from build123d import *

# Parameters (mm, degrees)
BOSS_EXTRUDE1_DEPTH = 12.7
SKETCH2_R           = 7.9375
CUT_EXTRUDE1_DEPTH  = 25.4
CUT_EXTRUDE2_DEPTH  = 15.24
CUT_EXTRUDE4_DEPTH  = 12.7
CUT_EXTRUDE3_DEPTH  = 12.7
FILLET4_R           = 3.81
CUT_EXTRUDE8_REACH  = 306.459
SKETCH10_R          = 3.302
CUT_EXTRUDE9_DEPTH  = 12.7
CUT_EXTRUDE10_DEPTH = 15.24
FILLET8_R           = 2.54
FILLET9_R           = 3.81
CUT_EXTRUDE11_DEPTH = 12.7
BOSS_EXTRUDE2_DEPTH = 12.7
SKETCH16_R          = 5.08
SKETCH16_R_2        = 2.54
BOSS_EXTRUDE3_DEPTH = 12.7
SKETCH17_R          = 2.54
CUT_EXTRUDE12_DEPTH = 12.7
CUT_EXTRUDE13_DEPTH = 12.7
BOSS_EXTRUDE4_DEPTH = 12.7


with BuildPart() as part:
    # Sketch1 → Boss-Extrude1 (new body)
    with BuildSketch(Plane.XY):
        with BuildLine():
            Line((22.605250022, 67.052290313), (98.805250022, 67.052290313))
            Line((98.805250022, 67.052290313), (98.805250022, 155.952290313))
            Line((98.805250022, 155.952290313), (-49.161223166, 287.699993186))
            ThreePointArc((-49.161223166, 287.699993186), (-96.236474745, 204.218681994), (-40.152034083, 126.502891159))
            Line((-40.152034083, 126.502891159), (22.605250022, 130.274128502))
            Line((22.605250022, 130.274128502), (22.605250022, 67.052290313))
        make_face()
    extrude(amount=BOSS_EXTRUDE1_DEPTH)

    # Sketch2 → Cut-Extrude1 (cut)
    with BuildSketch(Plane.XY.offset(12.7)):
        with Locations((-7.239749978, 209.038290313)):
            Circle(SKETCH2_R)
    extrude(amount=-CUT_EXTRUDE1_DEPTH, mode=Mode.SUBTRACT)

    # Sketch3 → Cut-Extrude2 (cut)
    with BuildSketch(Plane.XY.offset(12.7)):
        Polygon((41.655250022, 70.862290313), (41.655250022, 83.562290313), (60.705250022, 108.644790313), (79.755250022, 83.562290313), (79.755250022, 70.862290313), align=None)
        Polygon((26.415250022, 86.102290313), (39.115250022, 86.102290313), (57.847750022, 111.502290313), (39.115250022, 136.902290313), (26.415250022, 136.902290313), align=None)
        Polygon((94.995250022, 86.102290313), (82.295250022, 86.102290313), (63.562750022, 111.502290313), (82.295250022, 136.902290313), (94.995250022, 136.902290313), align=None)
        Polygon((41.655250022, 152.142290313), (41.655250022, 139.442290313), (60.705250022, 114.359790313), (79.755250022, 139.442290313), (79.755250022, 152.142290313), align=None)
    extrude(amount=-CUT_EXTRUDE2_DEPTH, mode=Mode.SUBTRACT)

    # Sketch5 → Cut-Extrude4 (cut)
    with BuildSketch(Plane.XY.offset(12.7)):
        with BuildLine():
            Line((-0.75941726, 237.80168728), (-42.818220106, 275.250377791))
            ThreePointArc((-42.818220106, 275.250377791), (-82.302366375, 205.259118271), (-35.720460653, 139.777057558))
            Line((-35.720460653, 139.777057558), (-14.124378137, 196.518923262))
            ThreePointArc((-14.124378137, 196.518923262), (-21.320643715, 206.617321953), (-17.910409102, 218.539326578))
            Line((-17.910409102, 218.539326578), (-0.75941726, 237.80168728))
        make_face()
        with BuildLine():
            Line((-5.26797782, 223.189077245), (3.983097906, 233.579004496))
            Line((3.983097906, 233.579004496), (15.365134305, 223.444565813))
            Line((15.365134305, 223.444565813), (6.380422315, 213.353792944))
            ThreePointArc((6.380422315, 213.353792944), (1.977645927, 219.954895508), (-5.26797782, 223.189077245))
        make_face()
        Polygon((20.700250022, 149.602290313), (-10.546123475, 195.20949671), (-35.128405597, 130.621646119), (20.700250022, 133.976525379), align=None)
    extrude(amount=-CUT_EXTRUDE4_DEPTH, mode=Mode.SUBTRACT)

    # Sketch4 → Cut-Extrude3 (cut)
    with BuildSketch(Plane.XY.offset(12.7)):
        Polygon((20.968161353, 155.952290313), (-3.903453401, 192.254898923), (20.952186028, 220.170386062), (68.306030681, 178.007049188), (68.306030681, 155.952290313), align=None)
        Polygon((91.166030681, 155.952290313), (70.846030681, 155.952290313), (70.846030681, 174.044992428), align=None)
    extrude(amount=-CUT_EXTRUDE3_DEPTH, mode=Mode.SUBTRACT)

    # Fillet4
    fillet4_edges = [part.edges().sort_by_distance(p)[0] for p in [
        (-10.546123475, 195.20949671, 6.35),
        (20.968161353, 155.952290313, 6.35),
    ]]
    fillet(fillet4_edges, radius=FILLET4_R)

    # Sketch10 → Cut-Extrude8 (cut, up to next)
    with BuildSketch(Plane.XY.offset(12.7), mode=Mode.PRIVATE) as cut_extrude8_sk1:
        with Locations((32.765250022, 77.212290313)):
            Circle(SKETCH10_R)
    cut_extrude8_tool1 = extrude(cut_extrude8_sk1.sketch, amount=-CUT_EXTRUDE8_REACH, mode=Mode.PRIVATE) & part.part
    # Sketch10 → Cut-Extrude8 (cut, up to next)
    with BuildSketch(Plane.XY.offset(12.7), mode=Mode.PRIVATE) as cut_extrude8_sk2:
        with Locations((32.765250022, 145.792290313)):
            Circle(SKETCH10_R)
    cut_extrude8_tool2 = extrude(cut_extrude8_sk2.sketch, amount=-CUT_EXTRUDE8_REACH, mode=Mode.PRIVATE) & part.part
    # Sketch10 → Cut-Extrude8 (cut, up to next)
    with BuildSketch(Plane.XY.offset(12.7), mode=Mode.PRIVATE) as cut_extrude8_sk3:
        with Locations((88.645250022, 145.792290313)):
            Circle(SKETCH10_R)
    cut_extrude8_tool3 = extrude(cut_extrude8_sk3.sketch, amount=-CUT_EXTRUDE8_REACH, mode=Mode.PRIVATE) & part.part
    # Sketch10 → Cut-Extrude8 (cut, up to next)
    with BuildSketch(Plane.XY.offset(12.7), mode=Mode.PRIVATE) as cut_extrude8_sk4:
        with Locations((88.645250022, 77.212290313)):
            Circle(SKETCH10_R)
    cut_extrude8_tool4 = extrude(cut_extrude8_sk4.sketch, amount=-CUT_EXTRUDE8_REACH, mode=Mode.PRIVATE) & part.part
    add(cut_extrude8_tool1.solids().sort_by_distance((32.76525, 77.21229, 12.7))[0], mode=Mode.SUBTRACT)
    add(cut_extrude8_tool2.solids().sort_by_distance((32.76525, 145.79229, 12.7))[0], mode=Mode.SUBTRACT)
    add(cut_extrude8_tool3.solids().sort_by_distance((88.64525, 145.79229, 12.7))[0], mode=Mode.SUBTRACT)
    add(cut_extrude8_tool4.solids().sort_by_distance((88.64525, 77.21229, 12.7))[0], mode=Mode.SUBTRACT)

    # Sketch11 → Cut-Extrude9 (cut)
    with BuildSketch(Plane.XY.offset(12.7)):
        with BuildLine():
            Line((-53.699981311, 142.099051734), (-44.964720503, 136.910524137))
            Line((-44.964720503, 136.910524137), (-50.020521881, 123.626837035))
            Line((-50.020521881, 123.626837035), (-66.867730014, 134.987909964))
            ThreePointArc((-66.867730014, 134.987909964), (-63.911601381, 136.652385518), (-60.829717039, 138.070540751))
            ThreePointArc((-60.829717039, 138.070540751), (-57.16682096, 139.911304034), (-53.699981311, 142.099051734))
        make_face()
    extrude(amount=-CUT_EXTRUDE9_DEPTH, mode=Mode.SUBTRACT)

    # Sketch13 → Cut-Extrude10 (cut)
    with BuildSketch(Plane.XY.offset(12.7)):
        with BuildLine():
            Line((-50.310364079, 281.9212995), (-42.818220106, 275.250377791))
            Line((-42.818220106, 275.250377791), (-55.824588323, 151.935966869))
            Line((-55.824588323, 151.935966869), (-61.138010202, 143.754384394))
            ThreePointArc((-61.138010202, 143.754384394), (-91.639185725, 215.652371712), (-50.310364079, 281.9212995))
        make_face()
    extrude(amount=-CUT_EXTRUDE10_DEPTH, mode=Mode.SUBTRACT)

    # Fillet8
    fillet8_edges = [part.edges().sort_by_distance(p)[0] for p in [
        (-60.829717039, 138.070540751, 6.35),
        (-61.138010202, 143.754384394, 6.35),
    ]]
    fillet(fillet8_edges, radius=FILLET8_R)

    # Fillet9
    fillet9_edges = [part.edges().sort_by_distance(p)[0] for p in [
        (-55.824588323, 151.935966869, 6.35),
    ]]
    fillet(fillet9_edges, radius=FILLET9_R)

    # Sketch14 → Cut-Extrude11 (cut)
    with BuildSketch(Plane.XY.offset(12.7)):
        Polygon((-0.75941726, 237.80168728), (-90.284904, 256.297301642), (-56.503441725, 294.237422972), (2.618728967, 241.595699413), align=None)
    extrude(amount=-CUT_EXTRUDE11_DEPTH, mode=Mode.SUBTRACT)

    # Sketch15 → Boss-Extrude2 (add)
    with BuildSketch(Plane.XY.offset(12.7)):
        Polygon((2.618728967, 241.595699413), (-83.695447283, 254.935945734), (-84.471371658, 249.915553183), (-1.404499457, 237.07719239), align=None)
    extrude(amount=-BOSS_EXTRUDE2_DEPTH)

    # Sketch16 → Boss-Extrude3 (add)
    with BuildSketch(Plane.XY.offset(12.7)):
        with Locations((-81.616731922, 249.474355701)):
            Circle(SKETCH16_R)
        with Locations((-81.616731922, 249.474355701)):
            Circle(SKETCH16_R_2, mode=Mode.SUBTRACT)
    extrude(amount=-BOSS_EXTRUDE3_DEPTH)

    # Sketch17 → Cut-Extrude12 (cut)
    with BuildSketch(Plane.XY.offset(12.7)):
        with Locations((-81.616731922, 249.474355701)):
            Circle(SKETCH17_R)
    extrude(amount=-CUT_EXTRUDE12_DEPTH, mode=Mode.SUBTRACT)

    # Sketch18 → Cut-Extrude13 (cut)
    with BuildSketch(Plane.XY.offset(12.7)):
        Polygon((-76.596339371, 248.698431326), (1.977645927, 219.954895508), (91.166030681, 155.952290313), (97.725254163, 155.952290313), (11.18255191, 258.990487802), (-76.596339371, 256.904187462), align=None)
    extrude(amount=-CUT_EXTRUDE13_DEPTH, mode=Mode.SUBTRACT)

    # Sketch20 → Boss-Extrude4 (add)
    with BuildSketch(Plane.XY.offset(12.7)):
        Polygon((90.745298735, 155.952290313), (-0.889749978, 217.928290313), (-76.596339371, 248.698431326), (-76.596339371, 253.838746498), (-2.444151583, 223.700375546), (97.725254163, 155.952290313), align=None)
    extrude(amount=-BOSS_EXTRUDE4_DEPTH)


solid = part.part
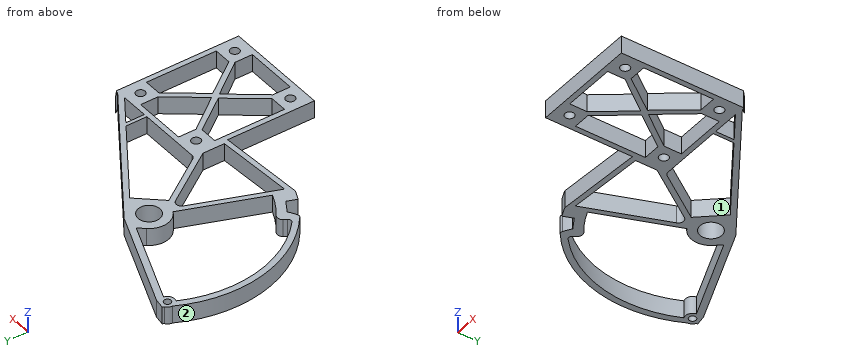
Geometry: final body of the model. Coordinates: model frame, mm. Face numbers are marked on the shaded views. Give positions to 0.01 mm unless a question says otherwise; leave off trailing zeros. Write each loop counter-clockwise with the first axis right and the second up, starting at its lowest first coordinate (ties: lowest second). Pieces come first, ordered by that corner, then holes. Notation, with made-up numbers: M -5.5,61 L 43.5,61 A25 cw 43.5,98 Z; hole C 67.5,0 d3. An arc over 180 degrees is marked long. Answer in a Markdown table with one row per item. Add a question column.
(1) Section D-D on x = 4. Return loops of the section in (y, z).
(2) Ray query, line 1 (Y direction, x = 91.5, z = 7.5); line 2 (Y direction, x = 5, z = 4); line 3 (Y direction, x = 48.5, z = 2). Return the intervals inside material, ascending.
(3) Section A-A on y = 119. Return loops of the section in (x, z), and give its area (3 significant figures).
(4) Section C-C on y = 229.5. Return loops of the section in (x, z), and give its area (3 significant figures).
(5) Mould query, pull axis X, two halves, no side actions, for the marked faces 1 and 2. Classes: +X half, -X half, draft (parallel to the pull), parting line (faces both ways), or undercut.
(6) Section B-B on x = -69. Return loops of the section in (y, z), and give its area (3 significant figures).
(7) First-contact query: pin 1 (4 mm diameter, centred on x = -81.62, y = 249.47, fed in from +Z); pin 2 (4 mm diameter, centred on x = 33.5, z = 5, fed in from +Y); pin 3 (7.5 mm diameter, centred on x = 32.77, y = 77.21, fed in from +Z); pin 4 (4 mm diameter, centred on x = 67, z = 9, fed in from +Y). Flat tips, straight axial feed; report the tip coordinate or a pass-through.
Result set:
| question | item | result |
|---|---|---|
| 1 | outline | M 129.16,0 L 132.97,0 L 132.97,12.7 L 129.16,12.7 Z; M 173.98,0 L 180.72,0 L 180.72,12.7 L 173.98,12.7 Z; M 201.13,0 L 219.34,0 L 219.34,12.7 L 201.13,12.7 Z |
| 2 | line 1 | y = 67.05 to 75.55, 78.87 to 86.1, 136.9 to 144.13, 147.45 to 160.16 |
| 2 | line 2 | y = 129.22 to 133.03, 172.52 to 179.26, 202.25 to 218.67 |
| 2 | line 3 | y = 67.05 to 70.86, 92.57 to 98.83, 124.18 to 130.43, 152.14 to 155.95, 184.52 to 189.25 |
| 3 | outline | M 22.61,0 L 26.42,0 L 26.42,12.7 L 22.61,12.7 Z; M 52.32,0 L 57.18,0 L 57.18,12.7 L 52.32,12.7 Z; M 64.23,0 L 69.09,0 L 69.09,12.7 L 64.23,12.7 Z; M 95,0 L 98.81,0 L 98.81,12.7 L 95,12.7 Z |
| 3 | area | 220 mm^2 |
| 4 | outline | M -94.02,0 L -89.39,0 L -89.39,12.7 L -94.02,12.7 Z; M -29.36,0 L -16.71,0 L -16.71,12.7 L -29.36,12.7 Z |
| 4 | area | 219 mm^2 |
| 5 | face 1 | undercut |
| 5 | face 2 | -X half |
| 6 | outline | M 145.01,0 L 151.14,0 L 151.14,12.7 L 145.01,12.7 Z; M 245.61,0 L 250.75,0 L 250.75,12.7 L 245.61,12.7 Z |
| 6 | area | 143 mm^2 |
| 7 | pin 1 | passes through |
| 7 | pin 2 | stops at y = 200.74 |
| 7 | pin 3 | stops at z = 12.7 |
| 7 | pin 4 | stops at y = 178.09 |
